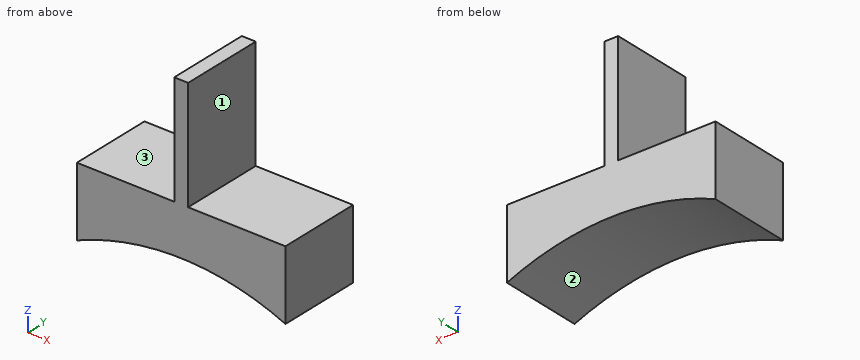
from build123d import *

# Parameters (mm, degrees)
F0_W     = 1
F0_H     = 8
F1_DEPTH = 6


with BuildPart() as f1:
    # F0 (on Front) → F1 (new body)
    with BuildSketch(Plane.XZ):
        with BuildLine():
            ThreePointArc((-7.5, 17.511496), (0, 19.05), (7.5, 17.511496))
            Line((7.5, 17.511496), (7.5, 22.511496))
            Line((7.5, 22.511496), (0.5, 22.511496))
            Line((0.5, 22.511496), (-0.5, 22.511496))
            Line((-0.5, 22.511496), (-7.5, 22.511496))
            Line((-7.5, 22.511496), (-7.5, 17.511496))
        make_face()
        with Locations((0, 26.511496)):
            Rectangle(F0_W, F0_H)
    extrude(amount=F1_DEPTH)


solid = f1.part
Model file for the job. Use its own axes, mm. Face numbers are marked on the shaded views. A direction names the side the tool comes from. Give positions to 0.01 mm unless a question says otherwise; leave off trailing zeros. Order: outer loops, then holes, each group sorted by start corner. A loop starts at its lowest first (then second) coordinate and runs counter-clockwise, first axis right, second up. Notation, with made-up numbers: (73.25, -17.75) - (87.25, -17.75) arc R29 cw to (87.25, 2.25) - close; hole circle Ø10 at (68.5, 82.25). An arc over 180 degrees is marked (long way). One line per item, written item: value.
Item 1: Pin check, flat tips, straight feed: pin 1 Ø1.5 at (x, y) = (-3.5, -4.5) entering from +Z; pin 2 Ø1.8 at (y, z) = (-1.5, 27.5) entering from +X; pin 3 Ø4 at (x, z) = (4.5, 24) entering from -Y; pin 4 Ø1 at (y, z) = (-3, 24.5) entering from -X. Stop position of each tip, or through.
Response values:
pin 1: z = 22.51
pin 2: x = 0.5
pin 3: y = -6
pin 4: x = -0.5
Item 2: Slice it at D-D (z = 29.5). List the corners of the cut face in (x, y).
Response values:
outline: (-0.5, -6) - (0.5, -6) - (0.5, 0) - (-0.5, 0) - close
Item 3: Tool access for the marked faces 1, 2 and 3: list every direction of +Z, -Z, +X, -X, +Y, -Y with a clear straight run to the whole face (end or side of a thin tool).
Response values:
face 1: +Z, +X, +Y, -Y
face 2: -Z, +Y, -Y
face 3: +Z, -X, +Y, -Y
Item 4: Slice it at B-B (z = 18.75). List the corners of the cut face in (x, y), then the cut area to 3 significant figures.
Response values:
outline: (-7.5, -6) - (-3.37, -6) - (-3.37, 0) - (-7.5, 0) - close; (3.37, -6) - (7.5, -6) - (7.5, 0) - (3.37, 0) - close
area: 49.6 mm2
Item 5: Wall check: line 1 (X direction, y = -1.7, z = 25.25); line 2 (Z direction, x = -0.25, y = -5.2); line 3 (Z direction, x = -0.75, y = -5.6). Give the ranges that are in metal, low to high.
Response values:
line 1: -0.5 to 0.5
line 2: 19.05 to 30.51
line 3: 19.04 to 22.51
Item 6: Slice it at C-C (x = 0). List the corners of the cut face in (y, z), then the cut area to 3 significant figures.
Response values:
outline: (-6, 19.05) - (0, 19.05) - (0, 30.51) - (-6, 30.51) - close
area: 68.8 mm2
Item 7: Slice it at A-A (y = -5). List the corners of the cut face in (x, z).
Response values:
outline: (-7.5, 17.51) arc R19.05 cw to (7.5, 17.51) - (7.5, 22.51) - (0.5, 22.51) - (0.5, 30.51) - (-0.5, 30.51) - (-0.5, 22.51) - (-7.5, 22.51) - close
